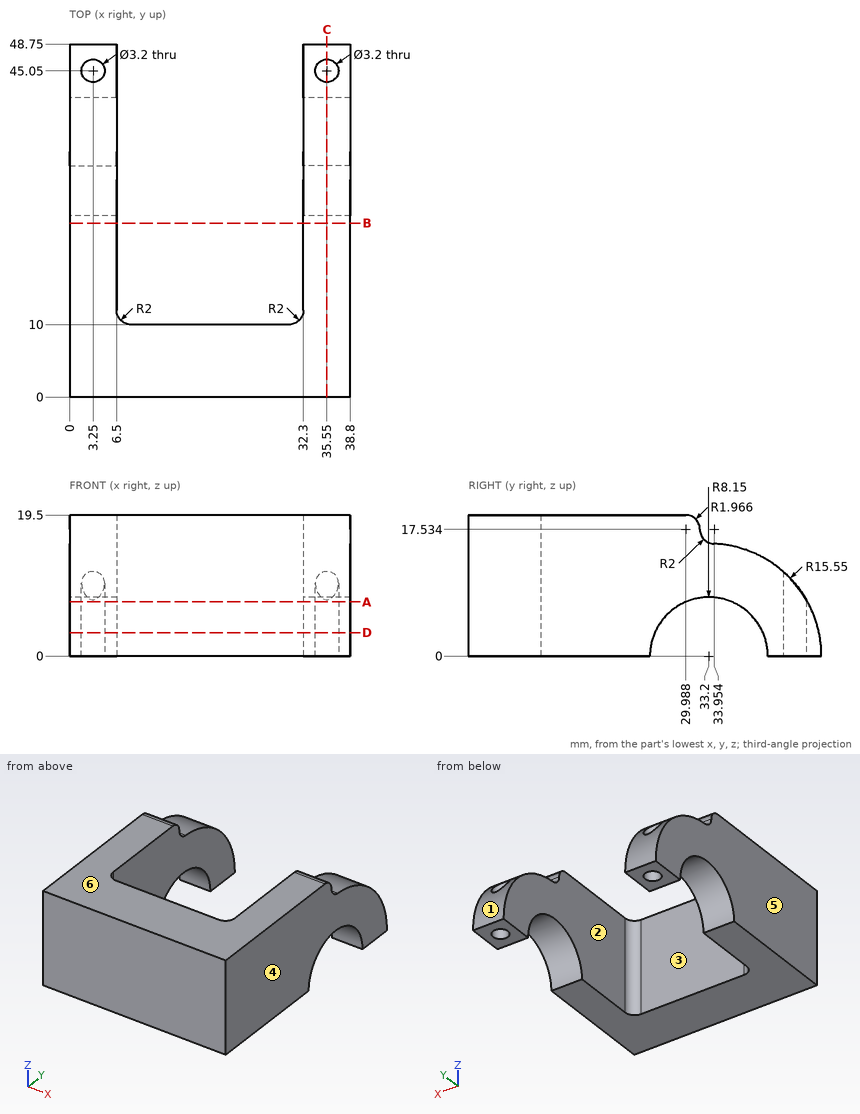
For this review, use the dimensioned drawing (mm, ordinates from the lowest corner) and the shaded views. A direction names the side the tool comes from. Give positions to 0.01 mm unless a question says otherwise; leave off trailing zeros. Order: outer loops, then holes, each group sorted by start corner. A loop starts at its lowest first (then second) coordinate and runs counter-clockwise, first axis right, second up.
1. For pin 1 Ø1.5 at (x, z) = (16.5, 13.5) entering from +Y; pin 2 Ø1.9 at (x, y) = (35.55, 45.05) entering from -Z, all flat-tipped, find the tip position at first contact; note any pin that passes through.
Solution:
pin 1: stops at y = 10
pin 2: passes through
2. Mouldability with a two-part tool opening along X and no side actions: class the marked faces 3, 4, 5 and 6 as +X half, -X half, draft (parallel to the pull), parting line (faces both ways), or undercut.
Solution:
face 3: undercut
face 4: +X half
face 5: -X half
face 6: draft
3. Add section D-D, the plane z = 3.25. State the section outline as (x, y) points.
Solution:
outline: (0, 0) - (38.8, 0) - (38.8, 25.73) - (32.3, 25.73) - (32.3, 12) arc R2 cw to (30.3, 10) - (8.5, 10) arc R2 cw to (6.5, 12) - (6.5, 25.73) - (0, 25.73) - close; (0, 40.67) - (6.5, 40.67) - (6.5, 48.41) - (0, 48.41) - close; (32.3, 40.67) - (38.8, 40.67) - (38.8, 48.41) - (32.3, 48.41) - close; hole circle Ø3.2 at (3.25, 45.05); hole circle Ø3.2 at (35.55, 45.05)
4. Tool access review of the marked faces 1 and 2: name each direction out of +Z, -Z, +X, -X, +Y, -Y from which nothing blocks a thin tool from reaching the whole face with its end or side.
Solution:
face 1: +Z, +X, -X, +Y
face 2: +Z, -Z, +Y
5. Add section B-B, the plane y = 24. State the section outline as (x, z) points.
Solution:
outline: (0, 0) - (6.5, 0) - (6.5, 19.5) - (0, 19.5) - close; (32.3, 0) - (38.8, 0) - (38.8, 19.5) - (32.3, 19.5) - close
6. To check wall thickness, follow L1, parallel to X at y = 30.5, z = 8.5; L2, parallel to Y at x = 26.5, z = 12.5; L3, parallel to Y at x = 35.55, z = 8.75. State the ranges of each line that lie inside material, in increasing order.
Solution:
L1: x = 0 to 6.5, 32.3 to 38.8
L2: y = 0 to 10
L3: y = 0 to 43.45
7. Add section C-C, the plane x = 35.55. State the section outline as (y, z) points, then the cut area to 3 significant figures.
Solution:
outline: (0, 0) - (25.05, 0) arc R8.15 cw to (41.35, 0) - (43.45, 0) - (43.45, 11.69) arc R15.55 ccw to (33.87, 15.54) arc R2 cw to (31.95, 17.53) arc R1.97 ccw to (29.99, 19.5) - (0, 19.5) - close; (46.65, 0) - (48.75, 0) arc R15.55 ccw to (46.65, 7.8) - close
area: 696 mm2
8. Add section A-A, the plane z = 7.5. State the section outline as (x, y) points, then the cut area to 3 significant figures.
Solution:
outline: (0, 0) - (38.8, 0) - (38.8, 30.01) - (32.3, 30.01) - (32.3, 12) arc R2 cw to (30.3, 10) - (8.5, 10) arc R2 cw to (6.5, 12) - (6.5, 30.01) - (0, 30.01) - close; (0, 36.39) - (6.5, 36.39) - (6.5, 46.82) - (0, 46.82) - close; (32.3, 36.39) - (38.8, 36.39) - (38.8, 46.82) - (32.3, 46.82) - close; hole circle Ø3.2 at (3.25, 45.05); hole circle Ø3.2 at (35.55, 45.05)
area: 769 mm2
